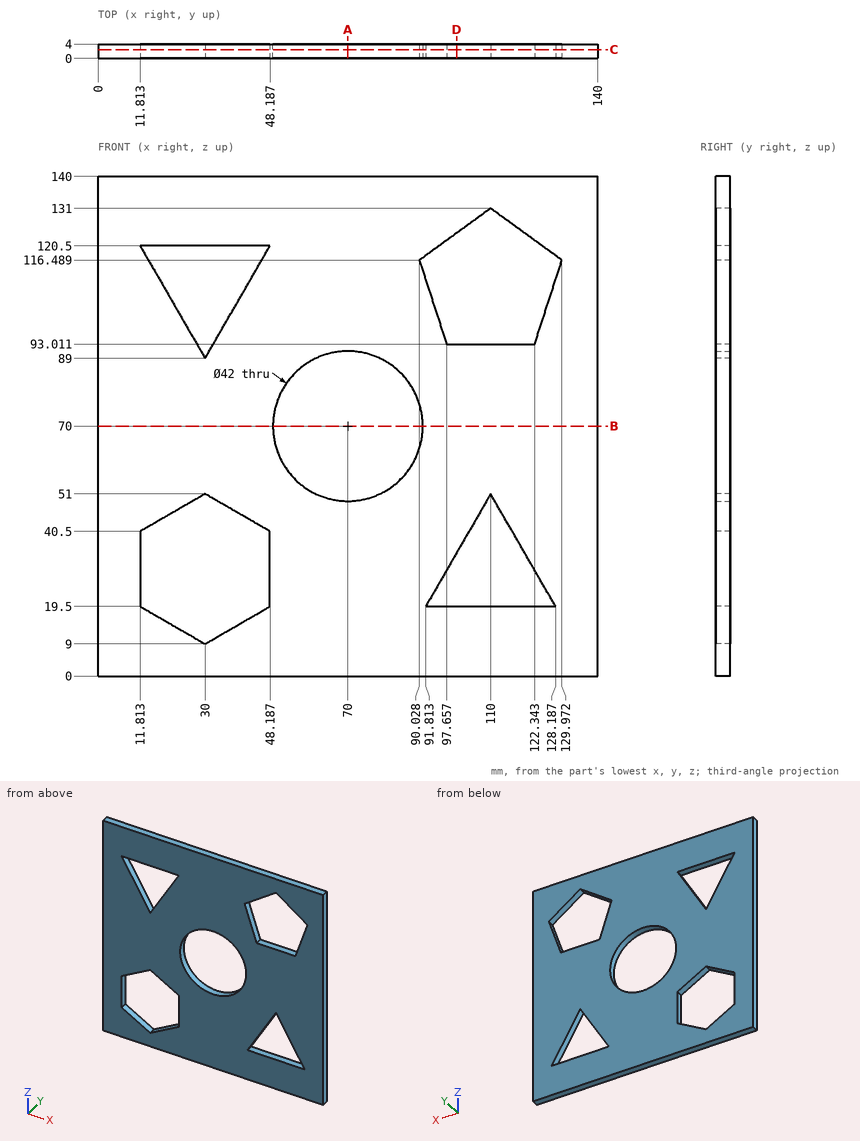
Geometry check sheet. Reference: drawing and pictorial views, mm from the part's lowest x, y, z. Give positions to 0.01 mm unless a question says otherwise; leave off trailing zeros. Order: outer loops, then holes, each group sorted by start corner. A loop starts at its lowest first (then second) coordinate and runs counter-clockwise, first axis right, second up.
1. Thickness scan on L1, parallel to Z at x = 70, y = 1.3; L2, parallel to Z at x = 104.5, y = 0.95 (1 decimal); L3, parallel to X at y = 2.7, z = 40.5 (1 decimal). Record the ranges inside material, lowest first.
2. Section check D-D, the plane x = 100.5. Enter the section's corners in (y, z) (1 decimal).
3. Section check B-B, the plane z = 70. Enter the section's corners in (x, y).
4. Gauge pin test, flat end, axial feed: pin 1 Ø1.5 at (y, z) = (0.5, 30) entering from -X. Record the tip position at first contact, or that the pin passes through.
5. Section check C-C, the plane y = 2.4. Enter the section's corners in (x, z).
6. Section check A-A, the plane x = 70. Enter the section's corners in (y, z), and give its area (3 significant figures).
Values follow:
1. L1: z = 0 to 49, 91 to 140
1. L2: z = 0 to 19.5, 41.5 to 93, 127 to 140
1. L3: x = 0 to 11.8, 48.2 to 103.9, 116.1 to 140
2. outline: (0, 0) - (4, 0) - (4, 19.5) - (0, 19.5) - close; (0, 34.5) - (4, 34.5) - (4, 93) - (0, 93) - close; (0, 124.1) - (4, 124.1) - (4, 140) - (0, 140) - close
3. outline: (0, 0) - (49, 0) - (49, 4) - (0, 4) - close; (91, 0) - (140, 0) - (140, 4) - (91, 4) - close
4. pin 1: stops at x = 0
5. outline: (0, 0) - (140, 0) - (140, 140) - (0, 140) - close; hole (11.81, 19.5) - (30, 9) - (48.19, 19.5) - (48.19, 40.5) - (30, 51) - (11.81, 40.5) - close; hole (11.81, 120.5) - (30, 89) - (48.19, 120.5) - close; hole circle Ø42 at (70, 70); hole (90.03, 116.49) - (97.66, 93.01) - (122.34, 93.01) - (129.97, 116.49) - (110, 131) - close; hole (91.81, 19.5) - (128.19, 19.5) - (110, 51) - close
6. outline: (0, 0) - (4, 0) - (4, 49) - (0, 49) - close; (0, 91) - (4, 91) - (4, 140) - (0, 140) - close
6. area: 392 mm2
